Answer from the drawing. Dimensions are ordinates in mm from the lowest x, y and z of the part. A direction names the side the tool comes from. Coordinates: 2 decimals unless noted, no trailing zeros. Loops run counter-clockwise (first coordinate to the right, second up) from the corner with the lowest first, then second, coordinate; pieces in that order, holes last. Notation, with made-up numbers: M -31,-9 L 24,-9 A9 ccw 24,5 Z; hole C 45.25,21.25 d11. An arc over 180 degrees is marked long. One line per item, written item: value. Start each with the question number.
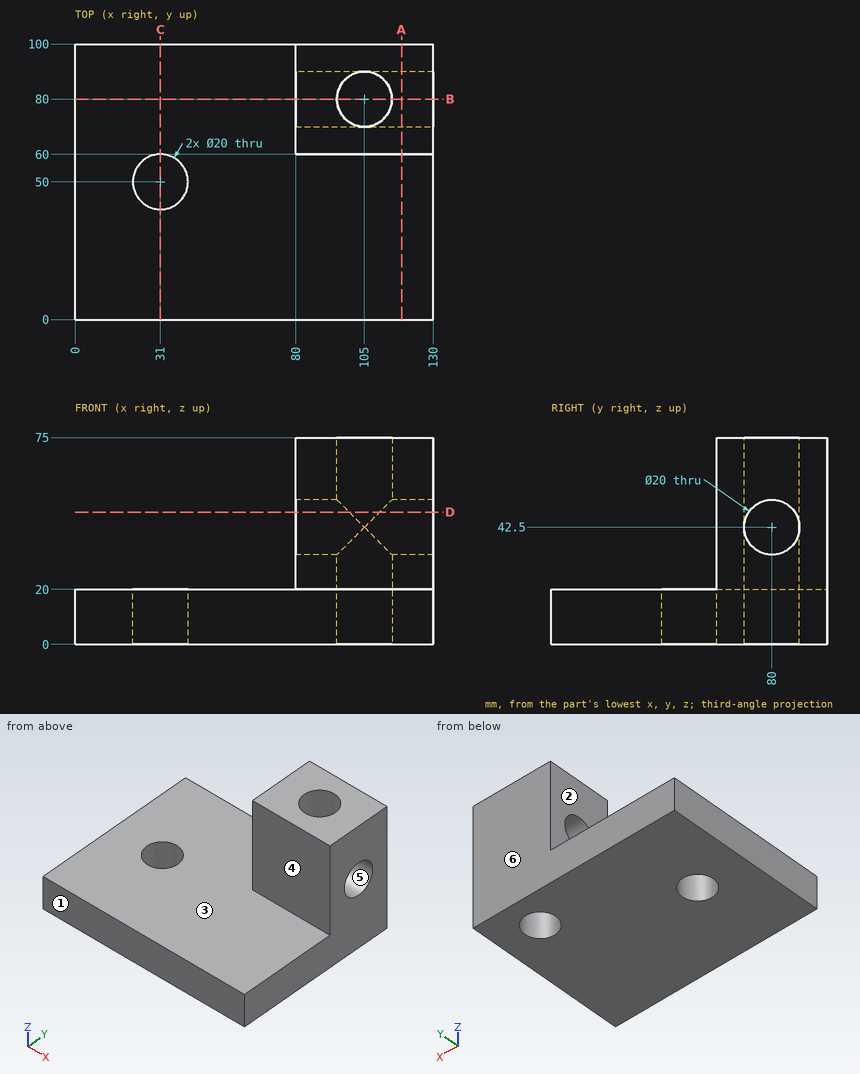
1) Section B-B (y = 80) is taken. Determine the outline of the cut face in (x, z), then the cut area to 3 significant figures.
2) Section D-D (z = 48) is taken. Determine the outline of the cut face in (x, y), then the cut area to 3 significant figures.
3) A tool of negligible diameter and unlimited length cuts with its end or side. For the marked faces 1, 2 and 3, from which of +Z, -Z, +X, -X, +Y, -Y can it reach the whole face along a straight path? Write none if from no direction.
4) Section C-C (x = 31) is taken. Determine the outline of the cut face in (y, z), then the cut area to 3 significant figures.
5) Consider line 1 along Y through (x, z) = (105, 68); line 2 along Y through (x, z) = (31, 9.75); line 3 along Z through (x, y) = (93.5, 80). Determine where each line is inside the solid, lowest interval first.
6) For a pull along Y with two mould halves and no side action, classify the marked faces 4, 5 and 6 as released by +Y, released by -Y, zero draft, split by the parting line, or undercut.
7) Flat-ended cylindrical pins translate along their axes: pin 1 (5 mm diameter, centred on x = 105.5, z = 58.5, fed in from -Y); pin 2 (10 mm diameter, centred on x = 43.5, y = 49.5, fed in from +Z). Find the tip coordinate at first contact, or state that the pin passes through.
8) Section A-A (x = 118.5) is taken. Determine the outline of the cut face in (y, z), then the cut area to 3 significant figures.
Results found:
1. outline: M 0,0 L 95,0 L 95,32.5 L 80,32.5 L 80,20 L 0,20 Z; M 80,52.5 L 95,52.5 L 95,75 L 80,75 Z; M 115,0 L 130,0 L 130,32.5 L 115,32.5 Z; M 115,52.5 L 130,52.5 L 130,75 L 115,75 Z
1. area: 3,250 mm²
2. outline: M 80,60 L 130,60 L 130,71.65 L 110.5,71.65 A10 cw 99.5,71.65 L 80,71.65 Z; M 80,88.35 L 99.5,88.35 A10 cw 110.5,88.35 L 130,88.35 L 130,100 L 80,100 Z
2. area: 1,140 mm²
3. face 1: +Z, -Z, +X, -X, -Y
3. face 2: +Z, -X, +Y, -Y
3. face 3: +Z, -X, -Y
4. outline: M 0,0 L 40,0 L 40,20 L 0,20 Z; M 60,0 L 100,0 L 100,20 L 60,20 Z
4. area: 1,600 mm²
5. line 1: y = 60 to 70, 90 to 100
5. line 2: y = 0 to 40, 60 to 100
5. line 3: z = 0 to 32.5, 52.5 to 75
6. face 4: released by -Y
6. face 5: undercut
6. face 6: released by +Y
7. pin 1: stops at y = 60
7. pin 2: stops at z = 20
8. outline: M 0,0 L 100,0 L 100,75 L 60,75 L 60,20 L 0,20 Z; hole C 80,42.5 d20
8. area: 3,890 mm²
